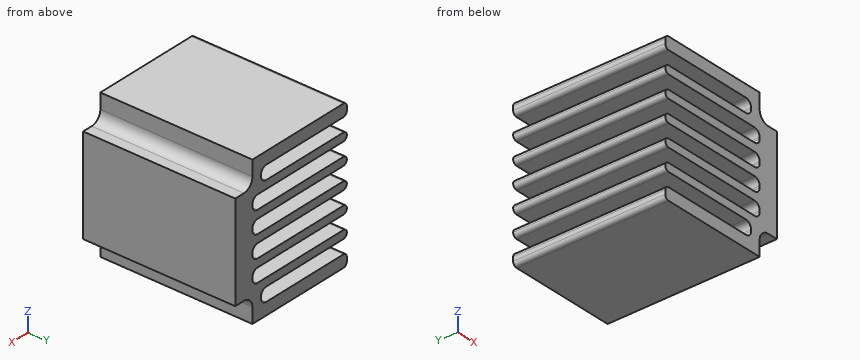
Autodesk Inventor part; units mm, degrees
ref_plane "YZ Plane" through (0, 0, 0) normal (1, 0, 0) x (0, 1, 0)
ref_plane "XZ Plane" through (0, 0, 0) normal (0, 1, 0) x (-1, 0, 0)
ref_plane "XY Plane" through (0, 0, 0) normal (0, 0, 1) x (1, 0, 0)
sketch "Skizze1" plane through (0, 0, 0) normal (0, 1, 0) x (-1, 0, 0)
  line L0 (6.5, 7.25) -> (-6.5, 7.25)
  line L1 (-6.5, 7.25) -> (-6.5, -7.25)
  line L2 (-6.5, -7.25) -> (6.5, -7.25)
  line L3 (6.5, -7.25) -> (6.5, 7.25)
  line L4 (6.5, 7.25) -> (-6.5, -7.25) construction
  line L5 (-6.5, 7.25) -> (6.5, -7.25) construction
  line L6 (-6.5, -7.25) -> (-4.5, -7.25)
  line L7 (-4.5, -7.25) -> (-4.5, -5.75)
  line L8 (-5.5, -4.75) -> (-6.5, -4.75)
  line L9 (-6.5, -4.75) -> (-6.5, -7.25)
  arc A0 (-4.5, -5.75) -> (-5.5, -4.75) centre (-5.5, -5.75) ccw
  line L10 (-6.5, 0) -> (-5.3357, 0)
  line L11 (6.5, -4.7) -> (-2.9, -4.7)
  line L12 (-3.5, -5.3) -> (-3.5, -5.45)
  line L13 (-2.9, -6.05) -> (6.5, -6.05)
  line L14 (6.5, -6.05) -> (6.5, -4.7)
  line L15 (6.5, -2.55) -> (-3.9, -2.55)
  line L16 (-4.5, -3.15) -> (-4.5, -3.3)
  line L17 (-3.9, -3.9) -> (6.5, -3.9)
  line L18 (6.5, -3.9) -> (6.5, -2.55)
  line L19 (6.5, -0.4) -> (-3.9, -0.4)
  line L20 (-4.5, -1) -> (-4.5, -1.15)
  line L21 (-3.9, -1.75) -> (6.5, -1.75)
  line L22 (6.5, -1.75) -> (6.5, -0.4)
  line L23 (-4.5, 7.25) -> (-4.5, 5.75)
  line L24 (-5.5, 4.75) -> (-6.5, 4.75)
  arc A1 (-5.5, 4.75) -> (-4.5, 5.75) centre (-5.5, 5.75) ccw
  line L25 (6.5, 4.7) -> (-2.9, 4.7)
  line L26 (-3.5, 5.3) -> (-3.5, 5.45)
  line L27 (-2.9, 6.05) -> (6.5, 6.05)
  line L28 (6.5, 2.55) -> (-3.9, 2.55)
  line L29 (-4.5, 3.15) -> (-4.5, 3.3)
  line L30 (-3.9, 3.9) -> (6.5, 3.9)
  line L31 (6.5, 0.4) -> (-3.9, 0.4)
  line L32 (-4.5, 1) -> (-4.5, 1.15)
  line L33 (-3.9, 1.75) -> (6.5, 1.75)
  arc A2 (-2.9, 6.05) -> (-3.5, 5.45) centre (-2.9, 5.45) ccw
  arc A3 (-3.5, 5.3) -> (-2.9, 4.7) centre (-2.9, 5.3) ccw
  arc A4 (-3.9, 3.9) -> (-4.5, 3.3) centre (-3.9, 3.3) ccw
  arc A5 (-4.5, 3.15) -> (-3.9, 2.55) centre (-3.9, 3.15) ccw
  arc A6 (-3.9, 1.75) -> (-4.5, 1.15) centre (-3.9, 1.15) ccw
  arc A7 (-4.5, 1) -> (-3.9, 0.4) centre (-3.9, 1) ccw
  arc A8 (-3.9, -0.4) -> (-4.5, -1) centre (-3.9, -1) ccw
  arc A9 (-4.5, -1.15) -> (-3.9, -1.75) centre (-3.9, -1.15) ccw
  arc A10 (-3.9, -2.55) -> (-4.5, -3.15) centre (-3.9, -3.15) ccw
  arc A11 (-4.5, -3.3) -> (-3.9, -3.9) centre (-3.9, -3.3) ccw
  arc A12 (-2.9, -4.7) -> (-3.5, -5.3) centre (-2.9, -5.3) ccw
  arc A13 (-3.5, -5.45) -> (-2.9, -6.05) centre (-2.9, -5.45) ccw
  point P0 (0, 0)
  point P1 (-4.5, -4.75)
  point P2 (-3.5, -6.05)
  point P3 (-3.5, -4.7)
  point P4 (-4.5, -3.9)
  point P5 (-4.5, -2.55)
  point P6 (-4.5, -1.75)
  point P7 (-4.5, -0.4)
  point P8 (-3.5, 6.05)
  point P9 (-3.5, 4.7)
  point P10 (-4.5, 3.9)
  point P11 (-4.5, 2.55)
  point P12 (-4.5, 1.75)
  point P13 (-4.5, 0.4)
  point P14 (6.5, -3.9)
  point P15 (6.5, -1.75)
  point P16 (6.5, 1.75)
  dimension "d0" = 13
  dimension "d1" = 14.5
  dimension "d2" = 2
  dimension "d3" = 2.5
  dimension "d4" = 1
  dimension "d5" = 10
  dimension "d6" = 1.35
  dimension "d7" = 11
  dimension "d8" = 1.35
  dimension "d9" = 1.2
  dimension "d10" = 0.8
  dimension "d11" = 11
  dimension "d12" = 1.35
  dimension "d13" = 0.8
  dimension "d14" = 0.8
  dimension "d15" = 0.6
extrude "Extrusion1" add sketch "Skizze1" along normal blind 15 contours L3 L27 A2 L26 A3 L25 L30 A4 L29 A5 L28 L33 A6 L32 A7 L31 L19 A8 L20 A9 L21 L15 A10 L16 A11 L17 L11 A12 L12 A13 L13 L2 L7 A0 L8 L1 L24 A1 L23 L0
fillet "Rundung1" radius 0.4 14 edges at (-6.5, 7.5, 4.7) (-6.5, 7.5, 3.9) (-6.5, 7.5, 2.55) (-6.5, 7.5, 1.75) (-6.5, 7.5, 0.4) (-6.5, 7.5, -0.4) (-6.5, 7.5, -1.75) (-6.5, 7.5, -2.55) (-6.5, 7.5, -3.9) (-6.5, 7.5, -4.7) (-6.5, 7.5, 7.25) (-6.5, 7.5, 6.05) (-6.5, 7.5, -6.05) (-6.5, 7.5, -7.25)
equation "\"d13\" = d10"
properties part number "Heatsink5160Pro"
The listing builds one solid part. Answer for the finished solid, in the listing's coordinates (mm). Coordinates: 2 decimals unless noted, no trailing zeros. Write each loop counter-clockwise with the first axis right and the second up, starting at its lowest first coordinate (ties: lowest second). Pieces come first, ordered by that corner, then holes. Notation, with made-up numbers: M 0.25,3 L 17.25,3 A30 ccw 17.25,34 Z; hole C 57,14 d9. An arc over 180 degrees is marked long. Put each result on its own line as item: value. Start each with the question number.
1. Consider line 1 (Z direction, x = 4, y = 12.5); line 2 (X direction, y = 11.75, z = -6.5); line 3 (X direction, y = 7.5, z = 1). Determine where each line is inside the solid, lowest interval first. Write a range as from..to.
2. Flat-ended cylindrical pins translate along their axes: P1, Ø1.6, axis at y = 4, z = -6.5, coming from the +X side; P2, Ø0.5, axis at x = 6, y = 10.5, coming from the +Z side. Find the tip coordinate at first contact, or state that the pin passes through.
3. A cutting plane is placed at A-A on x = -1. Write down the section's boundary in (y, z), then the cut area to 3 significant figures.
Resolved:
1. line 1: z = -7.25..-3.89, -2.56..-1.74, -0.41..0.41, 1.74..2.56, 3.89..7.25
1. line 2: x = -6.5..4.5
1. line 3: x = 4.5..6.5
2. P1: stops at x = 4.5
2. P2: stops at z = 4.75
3. outline: M 0,-7.25 L 15,-7.25 L 15,-6.05 L 0,-6.05 Z; M 0,-4.7 L 15,-4.7 L 15,-3.9 L 0,-3.9 Z; M 0,-2.55 L 15,-2.55 L 15,-1.75 L 0,-1.75 Z; M 0,-0.4 L 15,-0.4 L 15,0.4 L 0,0.4 Z; M 0,1.75 L 15,1.75 L 15,2.55 L 0,2.55 Z; M 0,3.9 L 15,3.9 L 15,4.7 L 0,4.7 Z; M 0,6.05 L 15,6.05 L 15,7.25 L 0,7.25 Z
3. area: 96.0 mm2
